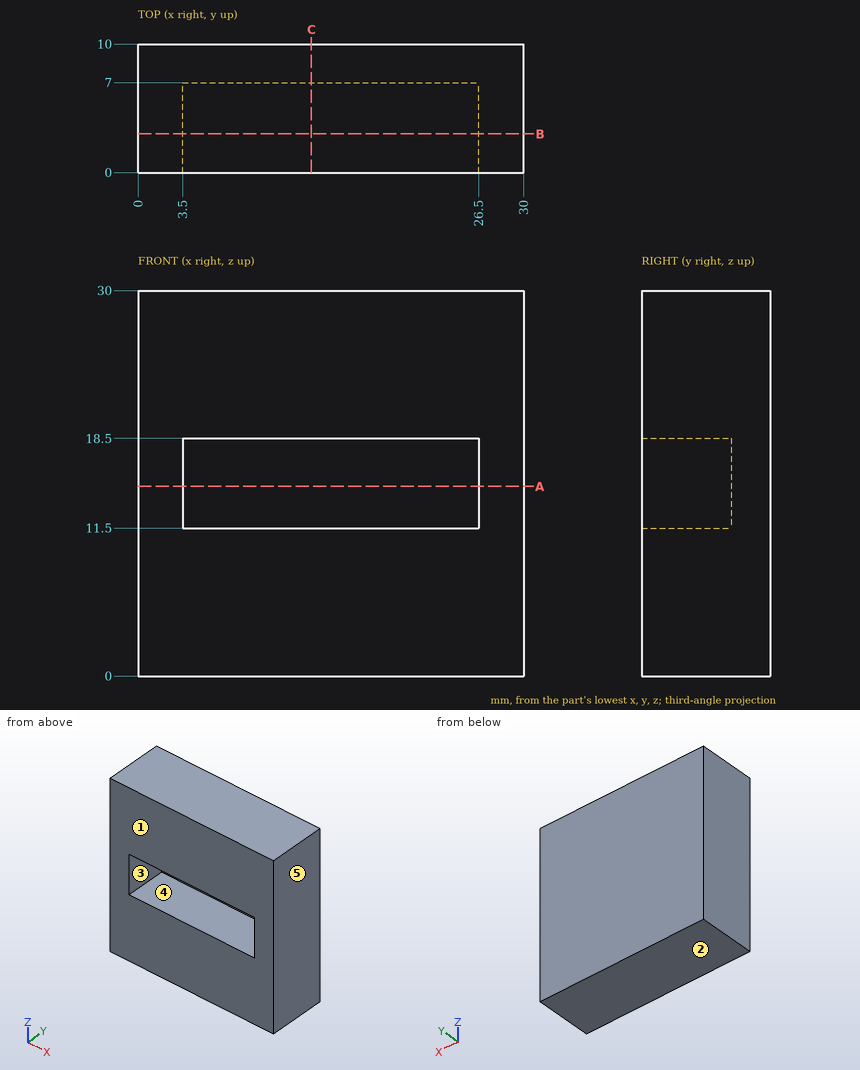
Here's the drawing with two shaded views (mm, measured from the low corner). I have some questions. A direction names the side the tool comes from. Coordinates: 2 decimals unless noted, no trailing zeros. Order: outer loops, then holes, each group sorted by start corner. A loop starts at its lowest first (then second) coordinate and runs counter-clockwise, first axis right, second up. Notation, with made-up numbers: (-29, 17.25) - (26, 17.25) arc R34 cw to (26, 52.25) - close; hole circle Ø9 at (-30, -24). An arc over 180 degrees is marked (long way). Answer in a Markdown table with one row per item.
1. For pin 1 (5.5 mm diameter, centred on y = 4.5, z = 15.5, fed in from -X); pin 2 (5.5 mm diameter, centred on x = 19, z = 15.5, fed in from -Y), each with a flat end and sliding along its axis, tell me the tip position at first contact or that it passes through.
Reply:
| item | result |
|---|---|
| pin 1 | stops at x = 0 |
| pin 2 | stops at y = 7 |
2. Suppose I cut it at C-C (x = 13.5). Please give me the cut outline in (y, z), and give its area (3 significant figures).
Reply:
| item | result |
|---|---|
| outline | (0, 0) - (10, 0) - (10, 30) - (0, 30) - (0, 18.5) - (7, 18.5) - (7, 11.5) - (0, 11.5) - close |
| area | 251 mm^2 |
3. Suppose I cut it at B-B (y = 3). Please give me the cut outline in (x, z).
Reply:
| item | result |
|---|---|
| outline | (0, 0) - (30, 0) - (30, 30) - (0, 30) - close; hole (3.5, 11.5) - (26.5, 11.5) - (26.5, 18.5) - (3.5, 18.5) - close |
4. For the marked faces 4 and 5, which set-ups out of +Z, -Z, +X, -X, +Y, -Y let a thin tool reach every point of the face, with its end or its side?
Reply:
| item | result |
|---|---|
| face 4 | -Y |
| face 5 | +Z, -Z, +X, +Y, -Y |
5. Suppose I cut it at A-A (z = 14.75). Please give me the cut outline in (x, y), and give its area (3 significant figures).
Reply:
| item | result |
|---|---|
| outline | (0, 0) - (3.5, 0) - (3.5, 7) - (26.5, 7) - (26.5, 0) - (30, 0) - (30, 10) - (0, 10) - close |
| area | 139 mm^2 |
6. If I drill on line 1 along Z through (x, y) = (23.5, 3.25); line 2 along Y through (x, z) = (24.5, 14.75), over which ranges is the centre line in solid material (lowest first)?
Reply:
| item | result |
|---|---|
| line 1 | z = 0 to 11.5, 18.5 to 30 |
| line 2 | y = 7 to 10 |
7. If we mould it in two halves opening along Z, with no side actions, what happens to the marked faces 1, 2 and 3? For each: pulls with the +Z half, pulls with the -Z half, needs draft (parallel to the pull), parting line crosses it, or undercut.
Reply:
| item | result |
|---|---|
| face 1 | needs draft |
| face 2 | pulls with the -Z half |
| face 3 | undercut |
